```python
from build123d import *

# Parameters (mm, degrees)
CUT_EXTRUDE1_DEPTH = 1.2
CUT_EXTRUDE1_DRAFT = -10
FILLET1_R          = 0.5


# Read off the part's stored shape, not the designer's step: LPattern1
with BuildPart() as part:
    # Sketch1 → Revolve1 (revolve)
    with BuildSketch(Plane.XY, mode=Mode.PRIVATE) as revolve1_sk:
        with BuildLine():
            Line((0, 1.8), (0, -4.8))
            Line((0, -4.8), (1.45, -4.8))
            Line((1.45, -4.8), (1.45, 0))
            Line((1.45, 0), (2.8, 0))
            ThreePointArc((2.8, 0), (2.941421356, 0.058578644), (3, 0.2))
            Line((3, 0.2), (3, 0.976556444))
            ThreePointArc((3, 0.976556444), (2.998479065, 1.001174742), (2.993939394, 1.025418612))
            ThreePointArc((2.993939394, 1.025418612), (2.630057903, 1.583487501), (2, 1.8))
            Line((2, 1.8), (0, 1.8))
        make_face()
    revolve(revolve1_sk.sketch.rotate(Axis((0, 1.8, 0), (0, -1, 0)), 180), axis=Axis((0, 1.8, 0), (0, -1, 0)))


with BuildPart() as cut_extrude1_tool:
    # Sketch2 → Cut-Extrude1 (with draft: the straight prism first)
    with BuildSketch(Plane(origin=(0, 1.8, 0), x_dir=(1, 0, 0), z_dir=(0, 1, 0))):
        Polygon((-0.5, 1.936491673), (-0.5, 0.5), (-1.936491673, 0.5), (-1.936491673, -0.5), (-0.5, -0.5), (-0.5, -1.936491673), (0.5, -1.936491673), (0.5, -0.5), (1.936491673, -0.5), (1.936491673, 0.5), (0.5, 0.5), (0.5, 1.936491673), align=None)
    extrude(amount=-CUT_EXTRUDE1_DEPTH)
    # Cut-Extrude1: the draft: its side faces are tilted about the plane it starts from
    cut_extrude1_sides = [cut_extrude1_tool.faces().sort_by_distance(p)[0] for p in [
        (-0.5, 1.2, -1.218245837),
        (-1.218245837, 1.2, -0.5),
        (-1.936491673, 1.2, 0),
        (-1.218245837, 1.2, 0.5),
        (-0.5, 1.2, 1.218245837),
        (0, 1.2, 1.936491673),
        (0.5, 1.2, 1.218245837),
        (1.218245837, 1.2, 0.5),
        (1.936491673, 1.2, 0),
        (1.218245837, 1.2, -0.5),
        (0.5, 1.2, -1.218245837),
        (0, 1.2, -1.936491673),
    ]]
    draft(cut_extrude1_sides, Plane(origin=(0, 1.8, 0), x_dir=(1, 0, 0), z_dir=(0, 1, 0)), CUT_EXTRUDE1_DRAFT)


with BuildPart() as part_1:
    add(part.part)

    # Cut-Extrude1: cut by cut_extrude1_tool
    add(cut_extrude1_tool.part, mode=Mode.SUBTRACT)

    # Fillet1
    fillet1_edges = [part_1.edges().sort_by_distance(p)[0] for p in [
        (0.394203812, 1.2, 0.394203812),
        (-0.394203812, 1.2, 0.394203812),
        (-0.394203812, 1.2, -0.394203812),
        (0.394203812, 1.2, -0.394203812),
    ]]
    fillet(fillet1_edges, radius=FILLET1_R)

    # Sketch3 → Cut-Revolve1 (revolve, cut)
    with BuildSketch(Plane.XY, mode=Mode.PRIVATE) as cut_revolve1_sk:
        Polygon((1.759807621, -4.65), (1.759807621, -4.95), (1.459807621, -4.95), (1.2, -4.8), (1.459807621, -4.65), align=None)
    revolve(cut_revolve1_sk.sketch.rotate(Axis((0, 0, 0), (0, -1, 0)), 180), axis=Axis((0, 0, 0), (0, -1, 0)), mode=Mode.SUBTRACT)

    # LPattern1 outline → LPattern1 (revolve, cut)
    with BuildSketch(Plane.XY):
        Polygon((1.45, -3.755662433), (1.2, -3.9), (1.45, -4.044337567), align=None)
        Polygon((1.2, -3.6), (1.45, -3.744337567), (1.45, -3.455662433), align=None)
        Polygon((1.45, -4.344337567), (1.45, -4.055662433), (1.2, -4.2), align=None)
        Polygon((1.2, -3.3), (1.45, -3.444337567), (1.45, -3.155662433), align=None)
        Polygon((1.45, -4.644337567), (1.45, -4.355662433), (1.2, -4.5), align=None)
        Polygon((1.2, -3), (1.45, -3.144337567), (1.45, -2.855662433), align=None)
        Polygon((1.2, -2.7), (1.45, -2.844337567), (1.45, -2.555662433), align=None)
        Polygon((1.2, -2.4), (1.45, -2.544337567), (1.45, -2.255662433), align=None)
        Polygon((1.2, -2.1), (1.45, -2.244337567), (1.45, -1.955662433), align=None)
        Polygon((1.2, -1.8), (1.45, -1.944337567), (1.45, -1.655662433), align=None)
        Polygon((1.2, -1.5), (1.45, -1.644337567), (1.45, -1.355662433), align=None)
        Polygon((1.2, -1.2), (1.45, -1.344337567), (1.45, -1.055662433), align=None)
        Polygon((1.2, -0.9), (1.45, -1.044337567), (1.45, -0.755662433), align=None)
        Polygon((1.2, -0.6), (1.45, -0.744337567), (1.45, -0.455662433), align=None)
        Polygon((1.2, -0.3), (1.45, -0.444337567), (1.45, -0.155662433), align=None)
    revolve(axis=Axis((0, 0, 0), (0, 1, 0)), mode=Mode.SUBTRACT)


solid = part_1.part
```
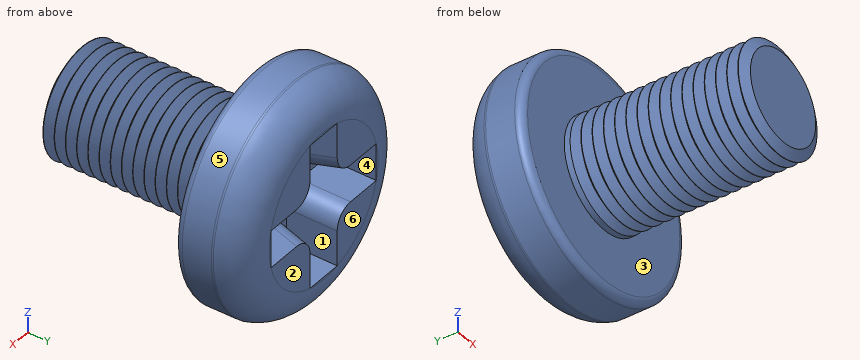
Model file for the job. Use its own axes, mm. Face numbers are marked on the shaded views. A direction names the side the tool comes from. Round coordinates to 2 decimals unless told otherwise and drop trailing zeros. Order: outer loops, then holes, each group sorted by start corner. A loop starts at its lowest first (then second) coordinate and runs counter-clockwise, first axis right, second up. Notation, with made-up numbers: (-1.75, 24) -> (31.25, 24) arc R25 ccw to (31.25, 54) -> close; hole circle Ø4 at (-21.75, 34). An arc over 180 degrees is marked (long way). Use one line per item in the form item = value.
Item 1: Pull direction X, two halves, no side cores. Call the marked faces 4, 5 and 6: released by +X, released by -X, zero draft, split by the parting line, or undercut.
Returned:
face_4 = undercut
face_5 = split by the parting line
face_6 = zero draft
Item 2: Drill centre lines: line 1 (Y direction, x = -0.75, z = 0); line 2 (Y direction, x = -0.5, z = -2); line 3 (X direction, y = 1, z = -1.75) (3 decimals). Where is each one in solid material? Low to high.
Returned:
line_1 = -4.8 to 0.6
line_2 = 0 to 1.8
line_3 = -2.435 to -0.359, 0.359 to 2.435
Item 3: Flat gauge pins, fed straight in: pin 1 Ø3 at (x, y) = (0.5, 1) entering from +Z; pin 2 Ø2 at (y, z) = (-0.5, 1.5) entering from +X. Where does each tip first touch, or does it go through?
Returned:
pin_1 = 3
pin_2 = 2.9
Item 4: Cut at A-A, the plane y = 0.5. Write the cut outline in (x, z), and give its area (3 significant figures).
Returned:
outline = circle Ø6 at (0, 0)
area = 28.3 mm^2
Item 5: Tool access for the marked faces 1, 2 and 3: list every direction of +Z, -Z, +X, -X, +Y, -Y with a clear straight run to the whole face (end or side of a thin tool).
Returned:
face_1 = +Y
face_2 = +Z, -Z, +X, -X, +Y
face_3 = -Y
